Here's how the part is built. I have some questions about the finished solid (model axes, mm). A direction names the side the tool comes from. Coordinates: 2 decimals unless noted, no trailing zeros. Write each loop counter-clockwise with the first axis right and the second up, starting at its lowest first coordinate (ties: lowest second). Pieces come first, ordered by that corner, then holes.
(1) Imagine slicing it at A-A, the plane x = 0. State how many separate pieces and enclosed holes the cut face has, plus the area to 3 significant figures.
(2) For pin 1 Ø3 at (y, z) = (2.5, -6) entering from +X; pin 2 Ø4 at (x, z) = (0, 0) entering from +Y; pin 3 Ø3 at (x, z) = (0, 9) entering from -Y; pin 4 Ø3 at (x, z) = (0.5, 1.5) entering from +Y, each with a flat end and sliding along its axis, tell me the tip position at first contact or that it passes through.
(3) Thinking about a two-plate mould opening in X: for faces 1 (the flat face through (-0.2, 0, 2.4)), 2 (the cylindrical face through (-11.99, 1.73, -0.53)), 3 (the cylindrical face through (7.4, 1.51, -0.07)), 4 (the cylindrical face through (-2.262, 4.268, 1.734)), which applies, released by +X, released by -X, zero draft, split by the parting line, or undercut?
(4) Please list where these lines run through material, in increasing order: probe 1 along Z at (x, y) = (9, 1.65); probe 2 along X at (y, z) = (4.6, 0); probe 3 along Y at (x, z) = (-3.5, -6.25).
(5) Imagine slicing it at B-B, the plane y = 3.3. List the corners of the cut face in (x, z) for me, plus the area to 3 significant figures.
(6) Which directions (+Z, -Z, +X, -X, +Y, -Y) give clear straight access to the entire face, cutting with the end or side of a thin tool? Please do faces 5 (the flat face through (0.1, 6, 3.5)), 6 (the flat face through (0, 3, 2)).
```python
from build123d import *

# Parameters (mm, degrees)
SKETCH2_R          = 1.6
CUT_EXTRUDE1_DEPTH = 4
CIRPATTERN1_COUNT  = 4
CHAMFER1_SIZE      = 0.5


with BuildPart() as part:
    # Sketch1 → Revolve1 (revolve)
    with BuildSketch(Plane.XY):
        Polygon((1.75, 0), (1.75, 3), (2.85, 3), (2.85, 6), (5.85, 6), (5.85, 3), (12, 3), (12, 0), align=None)
    revolve(axis=Axis((0, -26.625979541, 0), (0, 1, 0)))

    # Sketch2 → Cut-Extrude1 (cut, through all)
    with BuildSketch(Plane(origin=(0, 3, 0), x_dir=(1, 0, 0), z_dir=(0, 1, 0))):
        with Locations((9, 0)):
            Circle(SKETCH2_R)
    cut_extrude1 = extrude(amount=-CUT_EXTRUDE1_DEPTH, mode=Mode.SUBTRACT)

    # CirPattern1: Cut-Extrude1 ×4 about axis
    cirpattern1_axis = Axis((0, 0, 0), (0, 1, 0))
    for i in range(1, CIRPATTERN1_COUNT):
        add(cut_extrude1.rotate(cirpattern1_axis, i * 360 / CIRPATTERN1_COUNT), mode=Mode.SUBTRACT)

    # Chamfer1
    chamfer1_edges = [part.edges().sort_by_distance(p)[0] for p in [
        (7.4, 0, 0),
        (7.4, 3, 0),
        (0, 0, 7.4),
        (0, 3, 7.4),
        (-7.4, 0, 0),
        (-7.4, 3, 0),
        (0, 0, -7.4),
        (0, 3, -7.4),
        (-12, 0, 0),
        (-5.85, 6, 0),
        (-2.85, 6, 0),
        (-1.75, 0, 0),
    ]]
    chamfer(chamfer1_edges, length=CHAMFER1_SIZE)


solid = part.part
```
Recorded:
1. separate pieces: 4
1. enclosed holes: 0
1. area: 58.3 mm2
2. pin 1: stops at x = 11.12
2. pin 2: stops at y = 3
2. pin 3: passes through
2. pin 4: stops at y = 5.73
3. face 1: zero draft
3. face 2: split by the parting line
3. face 3: undercut
3. face 4: undercut
4. probe 1: z = -7.94 to -1.6, 1.6 to 7.94
4. probe 2: x = -5.85 to -2.85, 2.85 to 5.85
4. probe 3: y = 0 to 3
5. outline: circle Ø11.7 at (0, 0); hole circle Ø5.7 at (0, 0)
5. area: 82.0 mm2
6. face 5: +Z, -Z, +X, -X, +Y
6. face 6: +Y
